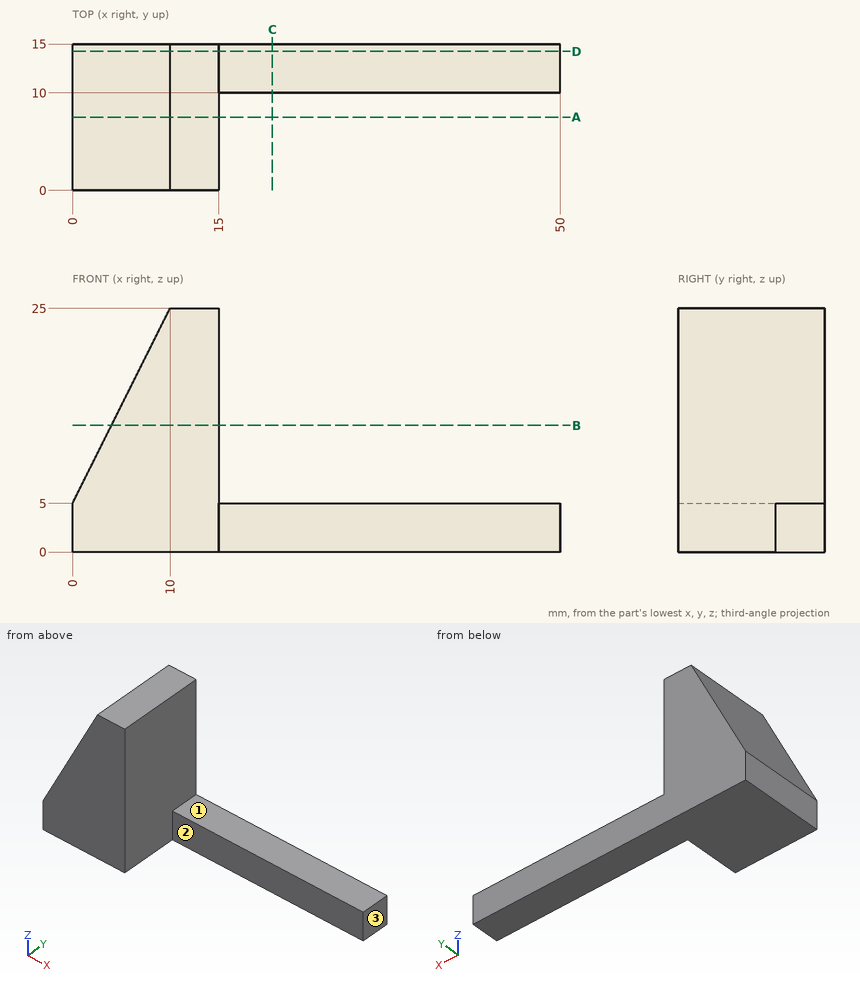
Geometry check sheet. Reference: drawing and pictorial views, mm from the part's lowest x, y, z. A direction names the side the tool comes from. Coordinates: 2 decimals unless noted, no trailing zeros. Order: outer loops, then holes, each group sorted by start corner. A loop starts at its lowest first (then second) coordinate and runs counter-clockwise, first axis right, second up. Notation, with made-up numbers: (-27, 21.5) - (20, 21.5) arc R18 ccw to (20, 33.5) - close; hole circle Ø4 at (71.5, 64). An arc over 180 degrees is marked (long way). One line per item, written item: value.
(1) Sectioned sample at A-A (y = 7.5). Enter the section's corners in (x, z).
Data:
outline: (0, 0) - (15, 0) - (15, 25) - (10, 25) - (0, 5) - close
(2) Sectioned sample at B-B (z = 13). Enter the section's corners in (x, y), and give its area (3 significant figures).
Data:
outline: (4, 0) - (15, 0) - (15, 15) - (4, 15) - close
area: 165 mm^2
(3) Thickness scan on probe 1 along Z at (x, y) = (46, 13); probe 2 along X at (y, z) = (1.5, 4.25); probe 3 along Y at (x, z) = (27, 3). Record the ranges inside material, lowest first. Write a range as from..to.
Data:
probe 1: z = 0..5
probe 2: x = 0..15
probe 3: y = 10..15
(4) Depth check by flat-ended pin: pin 1 Ø4 at (x, z) = (40, 2) entering from -Y; pin 2 Ø1.5 at (x, y) = (19.5, 11) entering from +Z; pin 3 Ø6 at (x, y) = (5, 12.5) entering from +Z. Enter the tip coordinate at first touch or a pass-through.
Data:
pin 1: stops at y = 10
pin 2: stops at z = 5
pin 3: stops at z = 21
(5) Sectioned sample at D-D (y = 14.25). Enter the section's corners in (x, z).
Data:
outline: (0, 0) - (50, 0) - (50, 5) - (15, 5) - (15, 25) - (10, 25) - (0, 5) - close
(6) Sectioned sample at C-C (x = 20.5). Enter the section's corners in (y, z), and give its area (3 significant figures).
Data:
outline: (10, 0) - (15, 0) - (15, 5) - (10, 5) - close
area: 25.0 mm^2
(7) Access from +Z, -Z, +X, -X, +Y, -Y to the whole of each face (thin tool, end or side, straight path). Record for the marked faces 1, 2 and 3.
Data:
face 1: +Z, +X, +Y, -Y
face 2: +Z, -Z, +X, -Y
face 3: +Z, -Z, +X, +Y, -Y
